Study the drawing (mm; zero at the part's minimum x, y, z) and answer. Round coordinates to 2 decimals unless told otherwise and drop trailing zeros. Write each loop counter-clockwise with the first axis right and the second up, starting at its lowest first coordinate (ties: lowest second). Pieces come first, ordered by that corner, then holes.
(1) A cutting plane is placed at B-B, the plane z = 0.7. Give the vertices of the cut face in (x, y), and give its area (3 significant figures).
(2) A cutting plane is placed at D-D, the plane x = 76. Give the vertices of the cut face in (y, z), and give its area (3 significant figures).
(3) Each of these flat-tipped pins is pushed along its axis until it touches: pin 1 Ø4.5 at (x, y) = (76, 4) entering from -Z; pin 2 Ø0.9 at (y, z) = (15, 1.5) entering from -X. Where does it stop, or does it pass through?
(4) Find the intervals of material crossed by probe 1 along Y at (x, z) = (76, 0.85); probe 2 along X at (y, z) = (21.5, 1.85); probe 3 along Y at (x, z) = (4, 0.7), in increasing order.
(5) A cutting plane is placed at A-A, the plane x = 4. Give the vertices of the cut face in (y, z), and give its area (3 significant figures).
(6) A cutting plane is placed at C-C, the plane y = 36. Give the vertices of the cut face in (x, z), and give its area (3 significant figures).
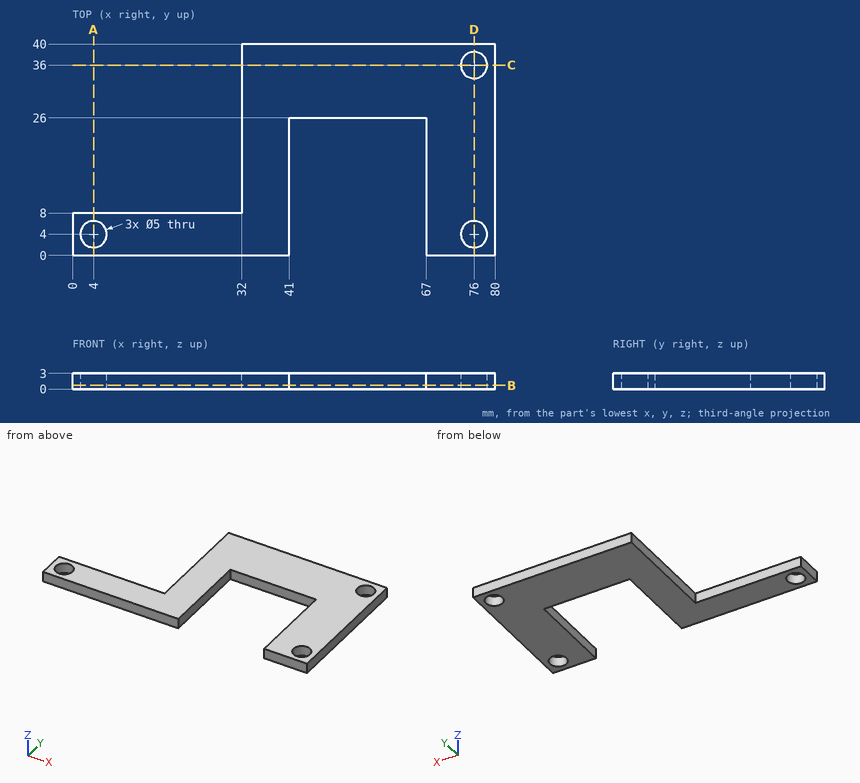
Solutions:
1. outline: (0, 0) - (41, 0) - (41, 26) - (67, 26) - (67, 0) - (80, 0) - (80, 40) - (32, 40) - (32, 8) - (0, 8) - close; hole circle Ø5 at (4, 4); hole circle Ø5 at (76, 4); hole circle Ø5 at (76, 36)
1. area: 1,440 mm2
2. outline: (0, 0) - (1.5, 0) - (1.5, 3) - (0, 3) - close; (6.5, 0) - (33.5, 0) - (33.5, 3) - (6.5, 3) - close; (38.5, 0) - (40, 0) - (40, 3) - (38.5, 3) - close
2. area: 90.0 mm2
3. pin 1: passes through
3. pin 2: stops at x = 32
4. probe 1: y = 0 to 1.5, 6.5 to 33.5, 38.5 to 40
4. probe 2: x = 32 to 41, 67 to 80
4. probe 3: y = 0 to 1.5, 6.5 to 8
5. outline: (0, 0) - (1.5, 0) - (1.5, 3) - (0, 3) - close; (6.5, 0) - (8, 0) - (8, 3) - (6.5, 3) - close
5. area: 9.00 mm2
6. outline: (32, 0) - (73.5, 0) - (73.5, 3) - (32, 3) - close; (78.5, 0) - (80, 0) - (80, 3) - (78.5, 3) - close
6. area: 129 mm2
